Build history of the part. All positions in model axes, mm. A direction names the side the tool comes from. Round coordinates to 2 decimals unless told otherwise and drop trailing zeros. Write each loop counter-clockwise with the first axis right and the second up, starting at its lowest first coordinate (ties: lowest second). Pieces come first, ordered by that corner, then holes. Notation, with made-up numbers: (37, 38) -> (57, 38) arc R18 cw to (57, 71) -> close; hole circle Ø6 at (31, 22). An arc over 180 degrees is marked (long way). Answer in a Markdown table with one row per item. Add a question column.
from build123d import *

# Parameters (mm, degrees)
F0_W      = 5.842
F0_H      = 12.7
F0_R      = 3.175
F2_DEPTH  = 3.175
F5_DEPTH  = 1.27
F4_R      = 1.524
F6_DEPTH  = 7.62
F10_R     = 1.524
F11_DEPTH = 17.78


# Not quite as in the source:
# - a feature of the source that left no trace in its solid (it failed there, or was rolled back) is left out


with BuildPart() as f1:
    # F0 (on Front) → F1 (revolve)
    with BuildSketch(Plane.XZ):
        Polygon((5.842, 12.7), (5.842, 0), (66.294, 0), (66.294, 12.7), (56.134, 12.7), (56.134, 10.16), (10.16, 10.16), (10.16, 12.7), align=None)
        with Locations((2.921, 6.35)):
            Rectangle(F0_W, F0_H)
    revolve(axis=Axis((33.147, 0, 0), (-1, 0, 0)))

    # F0 (on Front) → F2 (join, symmetric)
    with BuildSketch(Plane.XZ):
        with BuildLine():
            Line((5.842, 0), (0, 0))
            Line((0, 0), (-0.9398, 0))
            ThreePointArc((-0.9398, 0), (-3.1957909266, -4.5493385486), (-8.1826630726, -5.5069827884))
            Line((-8.1826630726, -5.5069827884), (5.842, -9.398))
            Line((5.842, -9.398), (5.842, 0))
        make_face()
        with BuildLine():
            Line((-0.9398, 0), (0, 0))
            Line((0, 0), (0, 12.7))
            Line((0, 12.7), (5.842, 12.7))
            Line((5.842, 12.7), (5.842, 15.24))
            Line((5.842, 15.24), (-0.508, 15.24))
            Line((-0.508, 15.24), (-10.8806298187, 3.8475430269))
            ThreePointArc((-10.8806298187, 3.8475430269), (-4.5919612295, 5.3297205562), (-0.9398, 0))
        make_face()
        with BuildLine():
            ThreePointArc((-8.1826630726, -5.5069827884), (-3.1957909266, -4.5493385486), (-0.9398, 0))
            ThreePointArc((-0.9398, 0), (-4.5919612295, 5.3297205562), (-10.8806298187, 3.8475430269))
            ThreePointArc((-10.8806298187, 3.8475430269), (-12.1459778134, -1.5837270034), (-8.1826630726, -5.5069827884))
        make_face()
        with Locations((-6.6548, 0)):
            Circle(F0_R, mode=Mode.SUBTRACT)
        with Locations((2.921, 6.35)):
            Rectangle(F0_W, F0_H)
    extrude(amount=F2_DEPTH, both=True)

    # F3: union 

    # F4 (on face) → F5 (join)
    with BuildSketch(Plane.YZ.offset(66.294)):
        with BuildLine():
            ThreePointArc((-5.08, 11.6397422652), (0, 12.7), (5.08, 11.6397422652))
            Line((5.08, 11.6397422652), (5.08, 15.24))
            Line((5.08, 15.24), (-5.08, 15.24))
            Line((-5.08, 15.24), (-5.08, 11.6397422652))
        make_face()
    extrude(amount=-F5_DEPTH)

    # F4 (on face) → F6 (join)
    with BuildSketch(Plane.YZ.offset(66.294)):
        with BuildLine():
            Line((5.08, 0), (5.08, 11.6397422652))
            ThreePointArc((5.08, 11.6397422652), (0, 12.7), (-5.08, 11.6397422652))
            Line((-5.08, 11.6397422652), (-5.08, 0))
            ThreePointArc((-5.08, 0), (0, 5.08), (5.08, 0))
        make_face()
        with BuildLine():
            ThreePointArc((-5.08, 11.6397422652), (0, 12.7), (5.08, 11.6397422652))
            Line((5.08, 11.6397422652), (5.08, 15.24))
            Line((5.08, 15.24), (-5.08, 15.24))
            Line((-5.08, 15.24), (-5.08, 11.6397422652))
        make_face()
        with BuildLine():
            ThreePointArc((-5.08, 0), (0, -5.08), (5.08, 0))
            ThreePointArc((5.08, 0), (0, 5.08), (-5.08, 0))
        make_face()
        Circle(F4_R, mode=Mode.SUBTRACT)
    extrude(amount=F6_DEPTH)

    # F7: union 

    # F10 (on face) → F11 (cut)
    with BuildSketch(Plane.XY.offset(15.24)):
        with Locations((2.667, 0)):
            Circle(F10_R)
    extrude(amount=-F11_DEPTH, mode=Mode.SUBTRACT)


solid = f1.part
(1) Mould opens along Z. For faces 5 (the face through (66.294, 0, 0)), 6 (the face through (3, 0, -2.54)), 7 (the face through (-4.149, -0.044, -6.626)) say: pulls with the +Z half, pulls with the -Z half, needs draft (parallel to the pull), parting line crosses it, or undercut.
(2) Probe line 1 along X through (y, z) = (-9.75, -8); line 2 along Z through (x, y) = (69, 0); line 3 along X through (y, z) = (-8.25, 4.75). List the from-to ranges inside material, lowest first.
(3) Saw through at D-D (y = 8.5). List the corners of the cut face in (x, z), plus the area to 3 significant figures.
(4) Saw through at B-B (y = -6). List the corners of the cut face in (x, z), plus the area to 3 significant figures.
(5) Drop flat-ended pins along their axis: P1, Ø2.5, axis at x = 71, z = 4.5, coming from the -Y side; P2, Ø7, axis at x = 69.5, z = 6, coming from the +Y side; P3, Ø2.5, axis at y = 0, z = 0, coming from the +X side; P4, Ø4, axis at x = 64, y = -6.5, coming from the +Z side. Give the stop position or say it passes through.
(6) Saw through at C-C (x = 17). List the corners of the cut face in (y, z).
(7) Which spindle directions (+Z, -Z, +X, -X, +Y, -Y) get a long thin tool onto all of the face, cutting with end or side? Do faces 1 (the face through (10.16, 9, 6)), 2 (the face through (70.05, -0.2, 1.51)), 3 (the face through (70.05, -0.11, -5.08)), 4 (the face through (4.12, 0.46, 6.47)). Say none if no direction does.
Answer sheet:
| question | item | result |
|---|---|---|
| 1 | face 5 | undercut |
| 1 | face 6 | pulls with the +Z half |
| 1 | face 7 | pulls with the -Z half |
| 2 | line 1 | x = 0 to 10.16, 56.13 to 66.29 |
| 2 | line 2 | z = -5.08 to -1.52, 1.52 to 15.24 |
| 2 | line 3 | x = 0 to 66.29 |
| 3 | outline | (0, -9.44) -> (10.16, -9.44) -> (10.16, -5.57) -> (56.13, -5.57) -> (56.13, -9.44) -> (66.29, -9.44) -> (66.29, 9.44) -> (56.13, 9.44) -> (56.13, 5.57) -> (10.16, 5.57) -> (10.16, 9.44) -> (0, 9.44) -> close |
| 3 | area | 895 mm² |
| 4 | outline | (0, -11.19) -> (10.16, -11.19) -> (10.16, -8.2) -> (56.13, -8.2) -> (56.13, -11.19) -> (66.29, -11.19) -> (66.29, 11.19) -> (56.13, 11.19) -> (56.13, 8.2) -> (10.16, 8.2) -> (10.16, 11.19) -> (0, 11.19) -> close |
| 4 | area | 1,210 mm² |
| 5 | P1 | stops at y = -5.08 |
| 5 | P2 | stops at y = 11.84 |
| 5 | P3 | stops at x = 66.29 |
| 5 | P4 | stops at z = 15.24 |
| 6 | outline | circle Ø20.32 at (0, 0) |
| 7 | face 1 | none |
| 7 | face 2 | +X |
| 7 | face 3 | -Z, +X |
| 7 | face 4 | +Z |
